Build history of the part. All positions in model axes, mm. A direction names the side the tool comes from. Round coordinates to 2 decimals unless told otherwise and drop trailing zeros. Order: outer loops, then holes, each group sorted by start corner. A loop starts at its lowest first (then second) coordinate and runs counter-clockwise, first axis right, second up. Notation, with made-up numbers: M 70.5,16.5 L 102.5,16.5 A9 cw 102.5,20.5 Z; hole C 77.25,66.25 d11. An arc over 180 degrees is marked long. One line per item, written item: value. Start each with the question number.
Item 1: Band-saw the part on C-C, the plane y = 3.5. Write the cut outline in (x, z), then the cut area to 3 significant figures.
Item 2: Band-saw the part on A-A, the plane z = 0. Write the cut outline in (x, y), then the cut area to 3 significant figures.
Item 3: Two-plate mould, pull along X, no slides. Class faces 1 (the flat face through (-9.3, 7, -2.7)), 2 (the cylindrical face through (10.74, 3.04, 2.38)), 3 (the cylindrical face through (-4.88, 6.85, -1.08)): +X half, -X half, draft (parallel to the pull), parting line (faces both ways), or undercut.
Item 4: Pin check, flat tips, straight feed: pin 1 (1 mm diameter, centred on x = -8.5, y = 5, fed in from -Z); pin 2 (3 mm diameter, centred on y = 3, z = 5, fed in from -X); pin 3 (2 mm diameter, centred on y = 2, z = 2, fed in from +X). Stop position of each tip, or through.
Item 5: Band-saw the part on D-D, the plane z = -9. Write the cut outline in (x, y), then the cut area to 3 significant figures.
Item 6: Probe L1, parallel to X at y = 6.8, z = 0; L2, parallel to Z at x = -3, y = 4.75; L3, parallel to Y at x = -8, z = -8. List the from-to ranges inside material, lowest first.
Item 7: Tool access for faces 4 (the cylindrical face through (3.905, 3.451, 0.867)), 5 (the flat face through (-4, 6.7, 4)), 6 (the flat face through (10, 6, 5)): list every direction of +Z, -Z, +X, -X, +Y, -Y with a clear straight run to the whole face (end or side of a thin tool).
Item 8: Band-saw the part on B-B, the plane x = 0. Write the cut outline in (y, z), then the cut area to 3 significant figures.
```python
from build123d import *

# Parameters (mm, degrees)
SKETCH2_R          = 9.5
SKETCH2_R_2        = 5
CUT_EXTRUDE1_DEPTH = 0.3
CUT_EXTRUDE2_START = -0.3
SKETCH3_R          = 9.5
SKETCH3_R_2        = 5
CUT_EXTRUDE2_DEPTH = 0.3


with BuildPart() as part:
    # Sketch1 → Revolve1 (revolve)
    with BuildSketch(Plane.XY, mode=Mode.PRIVATE) as revolve1_sk:
        Polygon((-12.5, 7), (-4, 7), (-4, 0), (-11, 0), (-11, 6), (-12.5, 6), align=None)
    revolve(revolve1_sk.sketch.rotate(Axis((0, 0, 0), (0, 1, 0)), 270), axis=Axis((0, 0, 0), (0, 1, 0)))

    # Sketch2 → Cut-Extrude1 (cut)
    with BuildSketch(Plane(origin=(0, 7, 0), x_dir=(1, 0, 0), z_dir=(0, 1, 0))):
        with Locations(Location((0, 0, 0), (0, 0, 270))):
            Circle(SKETCH2_R)
        with Locations(Location((0, 0, 0), (0, 0, 270))):
            Circle(SKETCH2_R_2, mode=Mode.SUBTRACT)
    extrude(amount=-CUT_EXTRUDE1_DEPTH, mode=Mode.SUBTRACT)

    # Sketch3 → Cut-Extrude2 (cut)
    with BuildSketch(Plane.XZ.offset(CUT_EXTRUDE2_START)):
        with Locations(Location((0, 0, 0), (0, 0, 90))):
            Circle(SKETCH3_R)
        with Locations(Location((0, 0, 0), (0, 0, 90))):
            Circle(SKETCH3_R_2, mode=Mode.SUBTRACT)
    extrude(amount=CUT_EXTRUDE2_DEPTH, mode=Mode.SUBTRACT)


solid = part.part
```
Output:
1. outline: C 0,0 d22; hole C 0,0 d8
1. area: 330 mm²
2. outline: M -12.5,6 L -11,6 L -11,0 L -9.5,0 L -9.5,0.3 L -5,0.3 L -5,0 L -4,0 L -4,7 L -5,7 L -5,6.7 L -9.5,6.7 L -9.5,7 L -12.5,7 Z; M 4,0 L 5,0 L 5,0.3 L 9.5,0.3 L 9.5,0 L 11,0 L 11,6 L 12.5,6 L 12.5,7 L 9.5,7 L 9.5,6.7 L 5,6.7 L 5,7 L 4,7 Z
2. area: 95.6 mm²
3. face 1: draft
3. face 2: parting line
3. face 3: undercut
4. pin 1: stops at z = -7.55
4. pin 2: stops at x = -10.43
4. pin 3: stops at x = 10.95
5. outline: M -8.67,6 L -6.32,6 L -6.32,0 L -3.04,0 L -3.04,0.3 L 3.04,0.3 L 3.04,0 L 6.32,0 L 6.32,6 L 8.67,6 L 8.67,7 L 3.04,7 L 3.04,6.7 L -3.04,6.7 L -3.04,7 L -8.67,7 Z
5. area: 89.6 mm²
6. L1: x = -12.5 to -9.5, -5 to -4, 4 to 5, 9.5 to 12.5
6. L2: z = -10.58 to -2.65, 2.65 to 10.58
6. L3: y = 6 to 7
7. face 4: +Y, -Y
7. face 5: +Y
7. face 6: -Y
8. outline: M 0,-11 L 6,-11 L 6,-12.5 L 7,-12.5 L 7,-9.5 L 6.7,-9.5 L 6.7,-5 L 7,-5 L 7,-4 L 0,-4 L 0,-5 L 0.3,-5 L 0.3,-9.5 L 0,-9.5 Z; M 0,4 L 7,4 L 7,5 L 6.7,5 L 6.7,9.5 L 7,9.5 L 7,12.5 L 6,12.5 L 6,11 L 0,11 L 0,9.5 L 0.3,9.5 L 0.3,5 L 0,5 Z
8. area: 95.6 mm²
